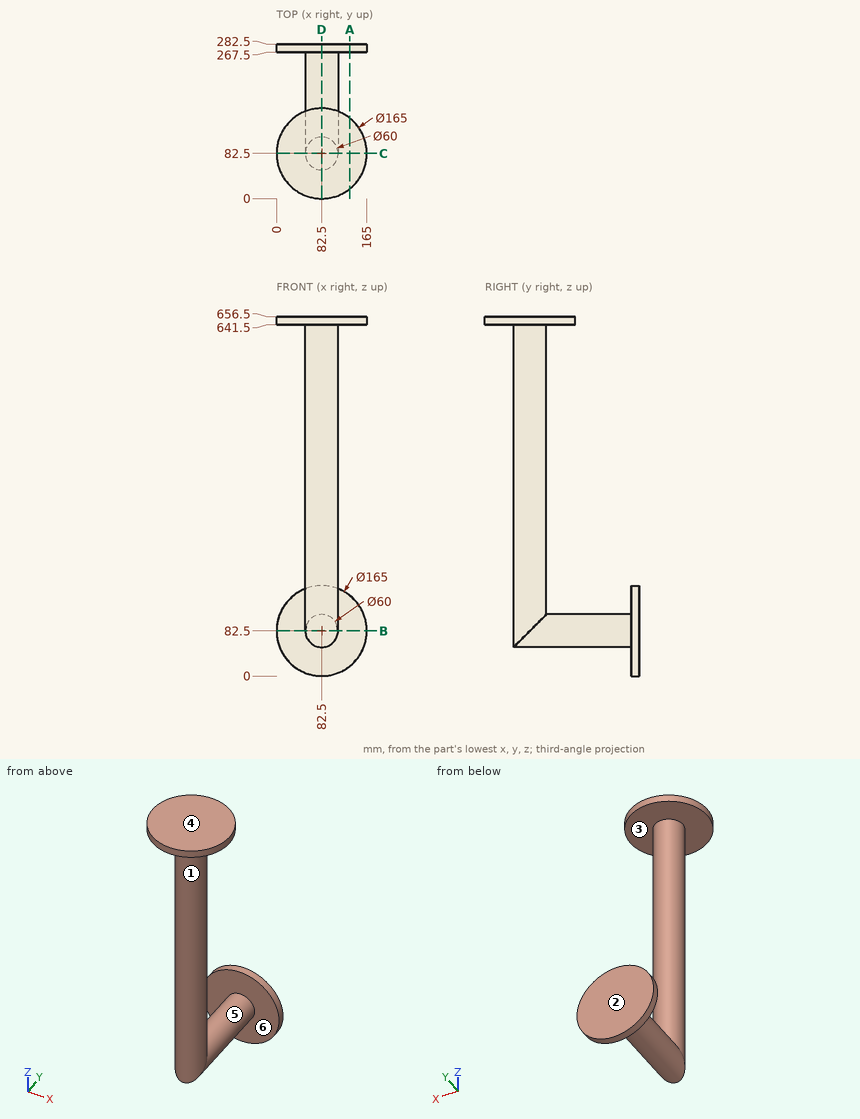
Source: three-view drawing plus pictorial views. Frame: mm from the lowest corner of the part. A direction names the side the tool comes from. Give positions to 0.01 mm unless a question says otherwise; leave off trailing zeros. Write each loop counter-clockwise with the first axis right and the second up, starting at its lowest first coordinate (ties: lowest second). Pieces come first, ordered by that corner, then holes. Notation, with made-up numbers: (49, 85.5) -> (102, 85.5) arc R15 ccw to (102, 91.5) -> close; hole circle Ø4 at (-2, 81.5). An arc over 180 degrees is marked (long way). Write item = value, one per line.
Q1. Cut plane A-A on x = 134. Return loops of the section in (y, z), then the cut area to 3 significant figures.
Here are the results:
outline = (18.05, 641.5) -> (146.95, 641.5) -> (146.95, 656.5) -> (18.05, 656.5) -> close; (267.5, 18.05) -> (282.5, 18.05) -> (282.5, 146.95) -> (267.5, 146.95) -> close
area = 3,870 mm²
Q2. Line query: line 1 (Z direction, x = 31, y = 37); line 2 (X direction, y = 229, z = 82); line 3 (Y direction, x = 22, z = 107.5). Output: solid intervals per line, ascending. Write a range as from..to.
Here are the results:
line_1 = 641.5..656.5
line_2 = 52.5..112.5
line_3 = 267.5..282.5
Q3. Mould query, pull axis Z, two halves, no side actions, for the marked faces 3, 4, 5 and 6. Classes: +Z half, -Z half, draft (parallel to the pull), parting line (faces both ways), or undercut.
Here are the results:
face_3 = undercut
face_4 = +Z half
face_5 = undercut
face_6 = draft
Q4. Reachability of the marked faces 1 and 2 from +Z, -Z, +X, -X, +Y, -Y: full face, straight path, thin tool, end or side. Return the list, or none.
Here are the results:
face_1 = none
face_2 = +Z, -Z, +X, -X, +Y
Q5. Cut plane D-D on x = 82.5. Return loops of the section in (y, z), then the cut area to 3 significant figures.
Here are the results:
outline = (0, 641.5) -> (52.5, 641.5) -> (52.5, 52.5) -> (267.5, 52.5) -> (267.5, 0) -> (282.5, 0) -> (282.5, 165) -> (267.5, 165) -> (267.5, 112.5) -> (112.5, 112.5) -> (112.5, 641.5) -> (165, 641.5) -> (165, 656.5) -> (0, 656.5) -> close
area = 49,600 mm²
Q6. First-contact query: pin 1 (1 mm diameter, centred on x = 83, z = 281, fed in from +Y); pin 2 (4 mm diameter, centred on x = 87, z = 361, fed in from -Y); pin 3 (12 mm diameter, centred on x = 84, y = 75.5, fed in from -Z). Flat tips, straight axial feed; report the tip coordinate or a pass-through.
Here are the results:
pin_1 = 112.5
pin_2 = 52.6
pin_3 = 52.5
Q7. Cut plane B-B on z = 82.5. Return loops of the section in (x, y), then the cut area to 3 significant figures.
Here are the results:
outline = (0, 267.5) -> (52.5, 267.5) -> (52.5, 82.5) arc R30 ccw to (112.5, 82.5) -> (112.5, 267.5) -> (165, 267.5) -> (165, 282.5) -> (0, 282.5) -> close
area = 15,000 mm²
Q8. Cut plane C-C on y = 82.5. Return loops of the section in (x, z).
Here are the results:
outline = (0, 641.5) -> (52.5, 641.5) -> (52.5, 82.5) arc R30 ccw to (112.5, 82.5) -> (112.5, 641.5) -> (165, 641.5) -> (165, 656.5) -> (0, 656.5) -> close
